from build123d import *

# Parameters (mm, degrees)
SKETCH1_R           = 1.7
BOSS_EXTRUDE1_DEPTH = 3
CHAMFER1_SIZE       = 5


with BuildPart() as part:
    # Sketch1 → Boss-Extrude1 (new body)
    with BuildSketch(Plane.XY):
        Polygon((-15, -25), (15, -25), (15, -15), (18, -15), (18, 15), (15, 15), (15, 25), (-15, 25), (-15, 15), (-21, 15), (-21, -15), (-15, -15), align=None)
        with Locations((11.5, -18)):
            Circle(SKETCH1_R, mode=Mode.SUBTRACT)
        with Locations((11.5, 18)):
            Circle(SKETCH1_R, mode=Mode.SUBTRACT)
        with Locations((-11.5, 18)):
            Circle(SKETCH1_R, mode=Mode.SUBTRACT)
        with Locations((-11.5, -18)):
            Circle(SKETCH1_R, mode=Mode.SUBTRACT)
    extrude(amount=BOSS_EXTRUDE1_DEPTH)

    # Chamfer1
    chamfer1_edges = [part.edges().sort_by_distance(p)[0] for p in [
        (-15, -25, 1.5),
        (-15, 25, 1.5),
    ]]
    chamfer(chamfer1_edges, length=CHAMFER1_SIZE)


solid = part.part
Geometry check sheet. Reference: the model listing, model coordinates, mm. A direction names the side the tool comes from. Round coordinates to 2 decimals unless told otherwise and drop trailing zeros. Loops run counter-clockwise (first coordinate to the right, second up) from the corner with the lowest first, then second, coordinate; pieces in that order, holes last. Notation, with made-up numbers: (-10.75, 57) - (0.25, 57) arc R33 cw to (0.25, 93) - close; hole circle Ø5 at (45.25, -32). An arc over 180 degrees is marked (long way). One line per question, with ' | ' between items. Start each with the question number.
1. Depth check by flat-ended pin: pin 1 (2.5 mm diameter, centred on x = -11.5, y = 18, fed in from +Z); pin 2 (0.9 mm diameter, centred on y = 17.5, z = 1.5, fed in from -X); pin 3 (0.9 mm diameter, centred on x = 17, z = 2, fed in from +Y); pin 4 (1.5 mm diameter, centred on x = -17.5, z = 1, fed in from -Y). Enter the tip coordinate at first touch or a pass-through.
2. Tool access check on faces 1 (the face through (15, -20, 1)), 2 (the face through (-15, -17, 1)), 3 (the face through (15, 20, 1)), 4 (the face through (-15, 18, 1)). Record the directions out of +Z, -Z, +X, -X, +Y, -Y that give a thin tool (end or side, any length) a straight path to the whole face; none if there is none.
3. Cross-section at B-B on z = 1.8. Record the cut outline in (x, y), then the cut area to 3 significant figures.
4. Cross-section at D-D on x = -16. Record the cut outline in (y, z), then the cut area to 3 significant figures.
5. Cross-section at C-C on y = 18. Record the cut outline in (x, z), then the cut area to 3 significant figures.
6. Cross-section at A-A on x = 11.5. Record the cut outline in (y, z), then the cut area to 3 significant figures.
7. Scan lines: line 1 (Y direction, x = 11.5, z = 1.45); line 2 (Y direction, x = 11, z = 1.6); line 3 (X direction, y = 16.5, z = 0.6). Record each from-to range of solid material in increasing order. Write a range as [from, to].
8. Draft check along X on faces 5 (the face through (18, 0, 1)), 6 (the face through (-2, 0, 3)), 7 (the face through (13.12, -17.49, 1.48)). Enter one of: released by +X, released by -X, zero draft, split by the parting line, or undercut.
Taken from the geometry:
1) pin 1: through | pin 2: x = -15 | pin 3: y = 15 | pin 4: y = -15
2) face 1: +Z, -Z, +X, -Y | face 2: +Z, -Z, -X, -Y | face 3: +Z, -Z, +X, +Y | face 4: +Z, -Z, -X, +Y
3) outline: (-21, -15) - (-15, -15) - (-15, -20) - (-10, -25) - (15, -25) - (15, -15) - (18, -15) - (18, 15) - (15, 15) - (15, 25) - (-10, 25) - (-15, 20) - (-15, 15) - (-21, 15) - close; hole circle Ø3.4 at (-11.5, -18); hole circle Ø3.4 at (-11.5, 18); hole circle Ø3.4 at (11.5, -18); hole circle Ø3.4 at (11.5, 18) | area: 1,710 mm²
4) outline: (-15, 0) - (15, 0) - (15, 3) - (-15, 3) - close | area: 90.0 mm²
5) outline: (-15, 0) - (-13.2, 0) - (-13.2, 3) - (-15, 3) - close; (-9.8, 0) - (9.8, 0) - (9.8, 3) - (-9.8, 3) - close; (13.2, 0) - (15, 0) - (15, 3) - (13.2, 3) - close | area: 69.6 mm²
6) outline: (-25, 0) - (-19.7, 0) - (-19.7, 3) - (-25, 3) - close; (-16.3, 0) - (16.3, 0) - (16.3, 3) - (-16.3, 3) - close; (19.7, 0) - (25, 0) - (25, 3) - (19.7, 3) - close | area: 130 mm²
7) line 1: [-25, -19.7], [-16.3, 16.3], [19.7, 25] | line 2: [-25, -19.62], [-16.38, 16.38], [19.62, 25] | line 3: [-15, -12.3], [-10.7, 10.7], [12.3, 15]
8) face 5: released by +X | face 6: zero draft | face 7: undercut
